Can you work these out from the model? Positions are in its coordinate system, mm. A direction names the side the tool comes from. Round coordinates to 2 decimals unless told otherwise and drop trailing zeros. Loops run counter-clockwise (first coordinate to the right, second up) from the corner with the lowest first, then second, coordinate; pieces in that order, holes last.
Autodesk Fusion 360 part; units mm, degrees
sketch "Sketch1" plane through (0, 0, 0) normal (0, 0, 1) x (1, 0, 0)
  line L0 (0, 0) -> (229, 0)
  line L1 (229, 0) -> (229, 146)
  line L2 (229, 146) -> (0, 146)
  line L3 (0, 146) -> (0, 0)
  dimension "d1" = 229
  dimension "d2" = 146
extrude "Extrude1" add sketch "Sketch1" along normal blind 20
sketch "Sketch2" plane through (0, 0, 20) normal (0, 0, 1) x (-1, 0, 0)
  line L0 (0, -146) -> (0, 0)
  line L1 (0, 0) -> (-229, 0)
  line L2 (-229, 0) -> (-229, -146)
  line L3 (-229, -146) -> (0, -146)
  line L4 (-3, -143) -> (-226, -143)
  line L5 (-226, -143) -> (-226, -3)
  line L6 (-226, -3) -> (-3, -3)
  line L7 (-3, -3) -> (-3, -143)
  dimension "d5" = 3
  dimension "d6" = 3
  dimension "d7" = 3
  dimension "d8" = 3
extrude "Extrude2" cut sketch "Sketch2" against normal blind 17 contours L4 L5 L6 L7
(1) If we section it at A-A, the plane z = 13.5: List the corners of the cut face in (x, y) for me.
Worked answers:
outline: (0, 0) - (229, 0) - (229, 146) - (0, 146) - close; hole (3, 3) - (226, 3) - (226, 143) - (3, 143) - close
(2) If I drill on line 1 (Y direction, x = 29.5, z = 18.25); line 2 (X direction, y = 71.5, z = 7.75); line 3 (Z direction, x = 13.5, y = 28), over which ranges is the centre line in solid material (lowest first)?
Worked answers:
line 1: y = 0 to 3, 143 to 146
line 2: x = 0 to 3, 226 to 229
line 3: z = 0 to 3
(3) Will these pins go through, and if not, where does the flat tip stop? P1, Ø5, axis at y = 46, z = 11, coming from the -X side; P2, Ø5, axis at x = 90.5, y = 67.5, coming from the +Z side.
Worked answers:
P1: stops at x = 0
P2: stops at z = 3
(4) If we mould it in two halves opening along X, with no side actions, what happens to faces 3 (the flat face through (229, 72, 10)), 4 (the flat face through (113, 74, 0)), 5 (the flat face through (113, 143, 12)), 6 (the flat face through (116, 72, 3))? For each: released by +X, released by -X, zero draft, split by the parting line, or undercut.
Worked answers:
face 3: released by +X
face 4: zero draft
face 5: undercut
face 6: undercut
(5) If we section it at B-B, the plane x = 107: List the corners of the cut face in (y, z) for me.
Worked answers:
outline: (0, 0) - (146, 0) - (146, 20) - (143, 20) - (143, 3) - (3, 3) - (3, 20) - (0, 20) - close
(6) If we section it at C-C, the plane y = 87: List the corners of the cut face in (x, z) for me, then the cut area to 3 significant figures.
Worked answers:
outline: (0, 0) - (229, 0) - (229, 20) - (226, 20) - (226, 3) - (3, 3) - (3, 20) - (0, 20) - close
area: 789 mm2
(7) For faces 1 (the flat face through (116, 3, 12)), 2 (the flat face through (116, 146, 10)), which set-ups out of +Z, -Z, +X, -X, +Y, -Y let a thin tool reach every point of the face, with its end or its side?
Worked answers:
face 1: +Z
face 2: +Z, -Z, +X, -X, +Y
